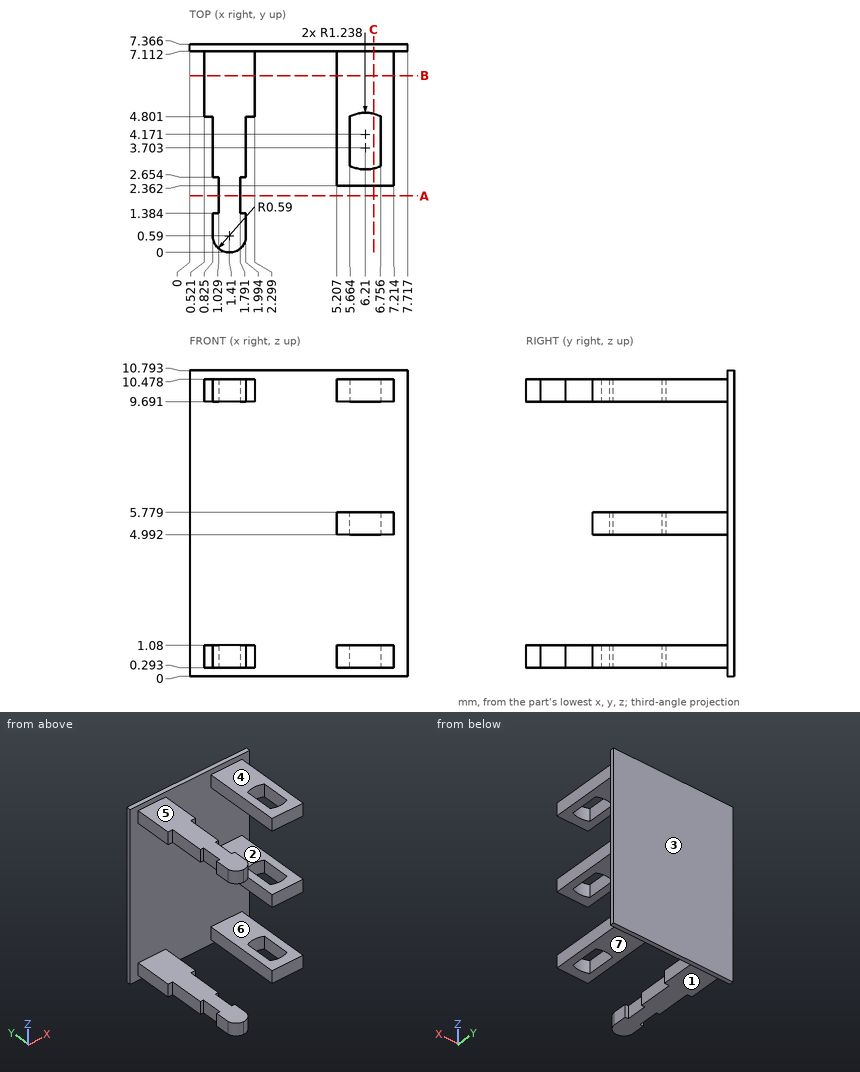
Study the drawing (mm; zero at the part's minimum x, y, z) and answer. A direction names the side the tool comes from. Round coordinates to 2 decimals unless told otherwise and drop trailing zeros. Loops run counter-clockwise (first coordinate to the right, second up) from the corner with the lowest first, then second, coordinate; pieces in that order, holes last.
Q1. Section C-C, the plane x = 6.5 is taken. Count the separate pieces of the cut face and the enclosed holes in it.
Q2. Given pin 1 Ø1 at (y, z) = (2.5, 1.5) entering from +X; pin 2 Ø2.5 at (x, z) = (4, 8) entering from -Y; pin 3 Ø3 at (x, y) = (2, 5) entering from +Z, each flat-ended and moving along its own axis, determine where each tip first touches the part or whether it passes through.
Q3. Find the intervals of material crossed by line 1 (X direction, y = 3.25, z = 1) (1 decimal); line 2 (Z direction, x = 5.25, y = 5.25); line 3 (Z direction, x = 1.5, y = 3.75), in increasing order.
Q4. Section A-A, the plane y = 2 is taken. Determine the outline of the cut face in (x, z).
Q5. Which of the six approach directions +Z, -Z, +X, -X, +Y, -Y give full straight-line access (tool end or side, diameter ignored) to the marked faces 5, 6 and 7?
Q6. Section B-B, the plane y = 6.25 is taken. Determine the outline of the cut face in (x, z).
Q7. For a pull along Z with two mould halves and no side action, classify the marked faces 1, 2, 3 and 4 as released by +Z, released by -Z, zero draft, split by the parting line, or undercut.
Completed:
1. separate pieces: 4
1. enclosed holes: 0
2. pin 1: stops at x = 7.21
2. pin 2: stops at y = 7.11
2. pin 3: stops at z = 10.48
3. line 1: x = 0.8 to 2, 5.2 to 5.7, 6.8 to 7.2
3. line 2: z = 0.29 to 1.08, 4.99 to 5.78, 9.69 to 10.48
3. line 3: z = 0.29 to 1.08, 9.69 to 10.48
4. outline: (1.03, 0.29) - (1.79, 0.29) - (1.79, 1.08) - (1.03, 1.08) - close; (1.03, 9.69) - (1.79, 9.69) - (1.79, 10.48) - (1.03, 10.48) - close
5. face 5: +Z, +X, -X, -Y
5. face 6: +X, -X, -Y
5. face 7: -Z, +X, -X, -Y
6. outline: (0.52, 0.29) - (2.3, 0.29) - (2.3, 1.08) - (0.52, 1.08) - close; (0.52, 9.69) - (2.3, 9.69) - (2.3, 10.48) - (0.52, 10.48) - close; (5.21, 0.29) - (7.21, 0.29) - (7.21, 1.08) - (5.21, 1.08) - close; (5.21, 4.99) - (7.21, 4.99) - (7.21, 5.78) - (5.21, 5.78) - close; (5.21, 9.69) - (7.21, 9.69) - (7.21, 10.48) - (5.21, 10.48) - close
7. face 1: released by -Z
7. face 2: undercut
7. face 3: zero draft
7. face 4: released by +Z
